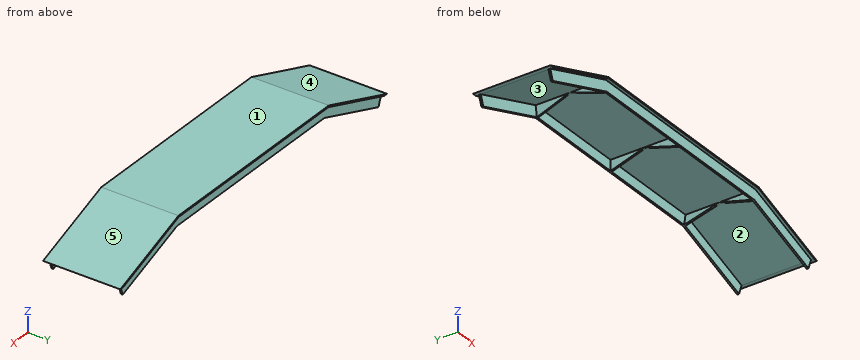
```python
from build123d import *

# Parameters (mm, degrees)
BOSS_EXTRUDE1_DEPTH = 109.600000002
BOSS_EXTRUDE2_DEPTH = 2.54
BOSS_EXTRUDE3_DEPTH = 2.54
RIB2_REACH          = 442.308
SKETCH5_WALL_W      = 932.98348183
SKETCH5_WALL_H      = 2.54
RIB3_REACH          = 442.308
SKETCH6_WALL_W      = 932.983481822
SKETCH6_WALL_H      = 2.54
RIB4_REACH          = 442.308
SKETCH7_WALL_W      = 932.98348183
SKETCH7_WALL_H      = 2.54
RIB5_REACH          = 442.308
SKETCH8_WALL_W      = 932.983481822
SKETCH8_WALL_H      = 2.54
RIB6_REACH          = 332.895
SKETCH13_WALL_W     = 714.088496324
SKETCH13_WALL_H     = 2.54
RIB7_REACH          = 332.895
SKETCH14_WALL_W     = 714.088496324
SKETCH14_WALL_H     = 2.54


with BuildPart() as part:
    # Sketch1 → Boss-Extrude1 (new body)
    with BuildSketch(Plane(origin=(0, 0, 0), x_dir=(1, 0, 0), z_dir=(0, 1, 0))):
        Polygon((-261, -120), (-150, -160), (150, -160), (261, -120), (266.899364373, -120), (150.349364373, -162), (-150.349364373, -162), (-266.899364373, -120), align=None)
    extrude(amount=BOSS_EXTRUDE1_DEPTH)

    # Sketch2 → Boss-Extrude2 (add)
    with BuildSketch(Plane(origin=(0, 4.249999882, 0), x_dir=(1, 0, 0), z_dir=(0, 1, 0))):
        Polygon((147.379767211, -145.000000028), (255.91470639, -105.888310234), (261, -120), (150, -160), (-150, -160), (-261, -120), (-255.91470639, -105.888310234), (-147.379767211, -145.000000028), align=None)
    extrude(amount=BOSS_EXTRUDE2_DEPTH)

    # Sketch4 → Boss-Extrude3 (add)
    with BuildSketch(Plane(origin=(0, 105.35000012, 0), x_dir=(1, 0, 0), z_dir=(0, 1, 0))):
        Polygon((-255.914706381, -105.888310207), (-147.379767206, -145), (147.379767206, -145), (255.914706381, -105.888310207), (261, -120), (150, -160), (-150, -160), (-261, -120), align=None)
    extrude(amount=-BOSS_EXTRUDE3_DEPTH)

    # Sketch5 wall → Rib2 (add, up to next)
    with BuildSketch(Plane(origin=(-148.689883603, 78.80500006, 152.5), x_dir=(-0.052022900314, -0.953205171679, 0.297814570709), z_dir=(0.164024260653, -0.302324164902, -0.938986763077)), mode=Mode.PRIVATE) as rib2_sk1:
        Rectangle(SKETCH5_WALL_W, SKETCH5_WALL_H)
    rib2_tool1 = extrude(rib2_sk1.sketch, amount=-RIB2_REACH, mode=Mode.PRIVATE) - part.part
    add(rib2_tool1.solids().sort_by_distance((-148.689883603, 78.80500006, 152.5))[0])

    # Sketch6 wall → Rib3 (add, up to next)
    with BuildSketch(Plane(origin=(-148.689883606, 30.794999942, 152.500000014), x_dir=(0.052022900223, -0.953205171842, -0.297814570204), z_dir=(0.164024260681, 0.302324164389, -0.938986763237)), mode=Mode.PRIVATE) as rib3_sk1:
        Rectangle(SKETCH6_WALL_W, SKETCH6_WALL_H)
    rib3_tool1 = extrude(rib3_sk1.sketch, amount=-RIB3_REACH, mode=Mode.PRIVATE) - part.part
    add(rib3_tool1.solids().sort_by_distance((-148.689883606, 30.794999942, 152.500000014))[0])

    # Sketch7 wall → Rib4 (add, up to next)
    with BuildSketch(Plane(origin=(148.689883603, 78.80500006, 152.5), x_dir=(0.052022900314, -0.953205171679, 0.297814570709), z_dir=(-0.164024260653, -0.302324164902, -0.938986763077)), mode=Mode.PRIVATE) as rib4_sk1:
        Rectangle(SKETCH7_WALL_W, SKETCH7_WALL_H)
    rib4_tool1 = extrude(rib4_sk1.sketch, amount=-RIB4_REACH, mode=Mode.PRIVATE) - part.part
    add(rib4_tool1.solids().sort_by_distance((148.689883603, 78.80500006, 152.5))[0])

    # Sketch8 wall → Rib5 (add, up to next)
    with BuildSketch(Plane(origin=(148.689883606, 30.794999942, 152.500000014), x_dir=(-0.052022900223, -0.953205171842, -0.297814570204), z_dir=(-0.164024260681, 0.302324164389, -0.938986763237)), mode=Mode.PRIVATE) as rib5_sk1:
        Rectangle(SKETCH8_WALL_W, SKETCH8_WALL_H)
    rib5_tool1 = extrude(rib5_sk1.sketch, amount=-RIB5_REACH, mode=Mode.PRIVATE) - part.part
    add(rib5_tool1.solids().sort_by_distance((148.689883606, 30.794999942, 152.500000014))[0])

    # Sketch13 wall → Rib6 (add, up to next)
    with BuildSketch(Plane(origin=(0, 78.80500006, 152.5), x_dir=(0, -0.954497664491, 0.298218390583), z_dir=(0, -0.298218390583, -0.954497664491)), mode=Mode.PRIVATE) as rib6_sk1:
        Rectangle(SKETCH13_WALL_W, SKETCH13_WALL_H)
    rib6_tool1 = extrude(rib6_sk1.sketch, amount=-RIB6_REACH, mode=Mode.PRIVATE) - part.part
    add(rib6_tool1.solids().sort_by_distance((0, 78.80500006, 152.5))[0])

    # Sketch14 wall → Rib7 (add, up to next)
    with BuildSketch(Plane(origin=(0, 30.794999942, 152.5), x_dir=(0, -0.954497664491, -0.298218390583), z_dir=(0, 0.298218390583, -0.954497664491)), mode=Mode.PRIVATE) as rib7_sk1:
        Rectangle(SKETCH14_WALL_W, SKETCH14_WALL_H)
    rib7_tool1 = extrude(rib7_sk1.sketch, amount=-RIB7_REACH, mode=Mode.PRIVATE) - part.part
    add(rib7_tool1.solids().sort_by_distance((0, 30.794999942, 152.5))[0])


solid = part.part
```
Geometry: final body of the model. Coordinates: model frame, mm. Face numbers are marked on the shaded views. A direction names the side the tool comes from. Coordinates: 2 decimals unless noted, no trailing zeros. Loops run counter-clockwise (first coordinate to the right, second up) from the corner with the lowest first, then second, coordinate; pieces in that order, holes last. Notation, with made-up numbers: (77, 21.5) -> (110, 21.5) arc R19 cw to (110, 55.5) -> close; hole circle Ø4 at (-26, 84.5). An arc over 180 degrees is marked (long way). Use a Markdown table: item, result. Add a question column.
(1) Line query: line 1 along Y through (x, z) = (242, 121); line 2 along Z through (x, y) = (128.5, 19.5); line 3 along Z through (x, y) = (207, 33.5). Output: solid intervals per line, ascending.
(2) Pin query (flat end, axial travel): pin 1 Ø3 at (x, y) = (-39.5, 104) entering from -Z; pin 2 Ø3 at (x, y) = (-158, 84) entering from +Z; pin 3 Ø6 at (x, y) = (106.5, 41) entering from -Z; pin 4 Ø16.5 at (x, z) = (-62.5, 153) entering from +Y. Return the tip coordinate at first contact, or that it passes through.
(3) Section query A-A, the plane x = 58. Return loops of the section in (y, z), plus the area to 3 significant figures.
(4) Section query C-C, the plane y = 93.5. Return loops of the section in (x, z), plus the area to 3 significant figures.
(5) Access query for the marked faces 1 and 2. Directions: +Z, -Z, +X, -X, +Y, -Y. A direction counts if a zero-diameter tool reaches every point of the face in a straight line with its end or side. Return the directions, or none.
(6) Mould query, pull axis X, two halves, no side actions, for the marked faces 3, 4 and 5. Classes: pulls with the +X half, pulls with the -X half, needs draft (parallel to the pull), parting line crosses it, or undercut.
(7) Section query B-B, the plane z = 114.5. Return loops of the section in (x, y).
(8) Section query D-D, the plane x = 219.5. Return loops of the section in (y, z), plus the area to 3 significant figures.
Answer:
| question | item | result |
|---|---|---|
| 1 | line 1 | y = 4.25 to 6.79, 102.81 to 105.35 |
| 1 | line 2 | z = 160 to 162 |
| 1 | line 3 | z = 139.46 to 141.59 |
| 2 | pin 1 | stops at z = 145 |
| 2 | pin 2 | stops at z = 159.78 |
| 2 | pin 3 | stops at z = 160 |
| 2 | pin 4 | stops at y = 109.6 |
| 3 | outline | (0, 160) -> (4.25, 160) -> (4.25, 145) -> (6.79, 145) -> (6.79, 160) -> (102.81, 160) -> (102.81, 145) -> (105.35, 145) -> (105.35, 160) -> (109.6, 160) -> (109.6, 162) -> (0, 162) -> close |
| 3 | area | 295 mm^2 |
| 4 | outline | (-266.9, 120) -> (-261, 120) -> (-151.21, 159.56) -> (-149.14, 147.69) -> (-146.64, 148.13) -> (-148.71, 160) -> (-1.27, 160) -> (-1.27, 147.91) -> (1.27, 147.91) -> (1.27, 160) -> (148.71, 160) -> (146.64, 148.13) -> (149.14, 147.69) -> (151.21, 159.56) -> (261, 120) -> (266.9, 120) -> (150.35, 162) -> (-150.35, 162) -> close |
| 4 | area | 1,180 mm^2 |
| 5 | face 1 | +Z, +X, -X, +Y, -Y |
| 5 | face 2 | -Z |
| 6 | face 3 | undercut |
| 6 | face 4 | pulls with the -X half |
| 6 | face 5 | pulls with the +X half |
| 7 | outline | (-259.02, 4.25) -> (-232.02, 4.25) -> (-232.02, 6.79) -> (-259.02, 6.79) -> close; (-259.02, 102.81) -> (-232.02, 102.81) -> (-232.02, 105.35) -> (-259.02, 105.35) -> close; (232.02, 4.25) -> (259.02, 4.25) -> (259.02, 6.79) -> (232.02, 6.79) -> close; (232.02, 102.81) -> (259.02, 102.81) -> (259.02, 105.35) -> (232.02, 105.35) -> close |
| 8 | outline | (0, 134.95) -> (4.25, 134.95) -> (4.25, 119.01) -> (6.79, 119.01) -> (6.79, 134.95) -> (102.81, 134.95) -> (102.81, 119.01) -> (105.35, 119.01) -> (105.35, 134.95) -> (109.6, 134.95) -> (109.6, 137.08) -> (0, 137.08) -> close |
| 8 | area | 314 mm^2 |
